Verification items for the finished model (mm, model axes). Face numbers are marked on the shaded views. A direction names the side the tool comes from. Round coordinates to 2 decimals unless told otherwise and drop trailing zeros. Order: outer loops, then holes, each group sorted by start corner. A loop starts at its lowest first (then second) coordinate and runs counter-clockwise, first axis right, second up.
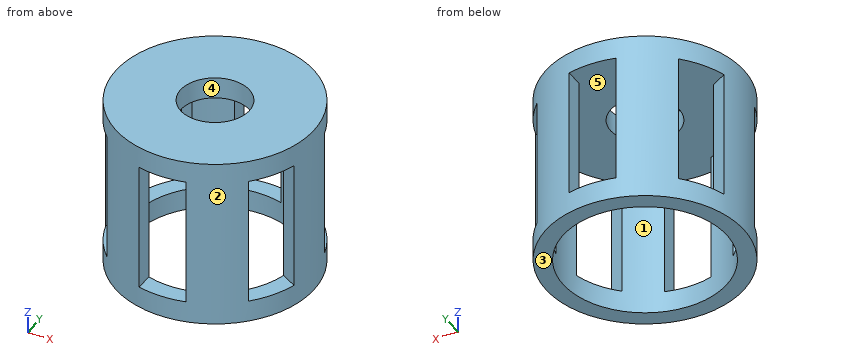
```python
from build123d import *

# Parameters (mm, degrees)
F0_R     = 11.5
F0_R_2   = 9.5
F1_DEPTH = 10
F2_W     = 5.4703750648
F2_H     = 6.3438538521
F3_DEPTH = 7.5
F4_R     = 4
F5_DEPTH = 2.5


with BuildPart() as f1:
    # F0 (on Top) → F1 (new body, symmetric)
    with BuildSketch(Plane.XY):
        Circle(F0_R)
        Circle(F0_R_2, mode=Mode.SUBTRACT)
    extrude(amount=F1_DEPTH, both=True)

    # F2 (on Top) → F3 (cut, symmetric)
    with BuildSketch(Plane.XY):
        with Locations((0, 9.139645283)):
            Rectangle(F2_W, F2_H)
        Polygon((-3.8006019335, 5.3526010656), (-9.2945405273, 8.5245279917), (-12.0297280597, 3.7870442173), (-6.5357894659, 0.6151172913), align=None)
        Polygon((-6.5357894659, -0.6151172913), (-12.0297280597, -3.7870442173), (-9.2945405273, -8.5245279917), (-3.8006019335, -5.3526010656), align=None)
        with Locations((0, -9.139645283)):
            Rectangle(F2_W, F2_H)
        Polygon((3.8006019335, -5.3526010656), (9.2945405273, -8.5245279917), (12.0297280597, -3.7870442173), (6.5357894659, -0.6151172913), align=None)
        Polygon((6.5357894659, 0.6151172913), (12.0297280597, 3.7870442173), (9.2945405273, 8.5245279917), (3.8006019335, 5.3526010656), align=None)
    extrude(amount=F3_DEPTH, both=True, mode=Mode.SUBTRACT)

    # F4 (on face) → F5 (join, through all)
    with BuildSketch(Plane(origin=(0, 0, 7.5), x_dir=(1, 0, 0), z_dir=(0, 0, -1))):
        with BuildLine():
            ThreePointArc((-2.7351875324, 9.0977331881), (-5.6685852928, -7.6234598955), (9.5, 0))
            ThreePointArc((9.5, 0), (7.6234598955, 5.6685852928), (2.7351875324, 9.0977331881))
            ThreePointArc((2.7351875324, 9.0977331881), (0, 9.5), (-2.7351875324, 9.0977331881))
        make_face()
        Circle(F4_R, mode=Mode.SUBTRACT)
    extrude(amount=-F5_DEPTH)


solid = f1.part
```
1) Go/stop test with flat-tipped pins: pin 1 Ø6.5 at (x, y) = (-2.5, 1) entering from -Z; pin 2 Ø11.5 at (x, y) = (0, 0) entering from +Z; pin 3 Ø2 at (x, z) = (-8, 1.5) entering from -Y; pin 4 Ø2.5 at (y, z) = (10.5, 1) entering from -X. Record where each tip stops, or that it passes through.
2) Scan lines: probe 1 along Z at (x, y) = (10.5, -4); probe 2 along Y at (x, z) = (0, 9.5); probe 3 along Z at (x, y) = (0.25, -5.5). Record each from-to range of solid material in increasing order.
3) Draft check along X on the marked faces 1, 2 and 3. Enter one of: released by +X, released by -X, zero draft, split by the parting line, or undercut.
4) Tool access check on the marked faces 4 and 5. Record the directions out of +Z, -Z, +X, -X, +Y, -Y that give a thin tool (end or side, any length) a straight path to the whole face; none if there is none.
5) Sectioned sample at D-D on z = 8. Record the cut outline in (x, y).
6) Sectioned sample at C-C on y = 0. Record the cut outline in (x, z).
7) Sectioned sample at B-B on x = 0. Record the cut outline in (y, z), then the cut area to 3 significant figures.
8) Sectioned sample at A-A on z = -6.25. Record the cut outline in (x, y).
Returned:
1. pin 1: stops at z = 7.5
1. pin 2: stops at z = 10
1. pin 3: stops at y = -9.12
1. pin 4: stops at x = -6.83
2. probe 1: z = -10 to -7.5, 7.5 to 10
2. probe 2: y = -11.5 to -4, 4 to 11.5
2. probe 3: z = 7.5 to 10
3. face 1: undercut
3. face 2: split by the parting line
3. face 3: zero draft
4. face 4: +Z, -Z
4. face 5: none
5. outline: circle Ø23 at (0, 0); hole circle Ø8 at (0, 0)
6. outline: (-11.5, -10) - (-9.5, -10) - (-9.5, 7.5) - (-4, 7.5) - (-4, 10) - (-11.5, 10) - close; (4, 7.5) - (9.5, 7.5) - (9.5, -10) - (11.5, -10) - (11.5, 10) - (4, 10) - close
7. outline: (-11.5, -10) - (-9.5, -10) - (-9.5, -7.5) - (-11.5, -7.5) - close; (-11.5, 7.5) - (-4, 7.5) - (-4, 10) - (-11.5, 10) - close; (4, 7.5) - (11.5, 7.5) - (11.5, 10) - (4, 10) - close; (9.5, -10) - (11.5, -10) - (11.5, -7.5) - (9.5, -7.5) - close
7. area: 47.5 mm2
8. outline: (-11.04, -3.22) - (-9.25, -2.18) arc R9.5 cw to (-9.25, 2.18) - (-11.04, 3.22) arc R11.5 ccw to start; (-8.31, -7.95) arc R11.5 ccw to (-2.74, -11.17) - (-2.74, -9.1) arc R9.5 cw to (-6.51, -6.92) - close; (-8.31, 7.95) - (-6.51, 6.92) arc R9.5 cw to (-2.74, 9.1) - (-2.74, 11.17) arc R11.5 ccw to start; (2.74, -11.17) arc R11.5 ccw to (8.31, -7.95) - (6.51, -6.92) arc R9.5 cw to (2.74, -9.1) - close; (2.74, 9.1) arc R9.5 cw to (6.51, 6.92) - (8.31, 7.95) arc R11.5 ccw to (2.74, 11.17) - close; (9.25, -2.18) - (11.04, -3.22) arc R11.5 ccw to (11.04, 3.22) - (9.25, 2.18) arc R9.5 cw to start
